Can you work these out from the model? Positions are in its coordinate system, mm. Coordinates: 2 decimals unless noted, no trailing zeros. Order: outer loops, then holes, each group sorted by start corner. A loop starts at its lowest first (then second) coordinate and runs counter-clockwise, first axis right, second up. Notation, with made-up numbers: M -6,23.5 L 48,23.5 A22 ccw 48,58.5 Z; hole C 5.25,-27.5 d1. An arc over 180 degrees is marked long. Answer as a JSON object with one key per item and string values.
Autodesk Inventor part; units mm, degrees
ref_plane "Work Plane1" through (15, -19.5, -83) normal (0, 0, -1) x (0, 1, 0)
ref_plane "YZ Plane" through (0, 0, 0) normal (1, 0, 0) x (0, 1, 0)
ref_plane "XZ Plane" through (0, 0, 0) normal (0, 1, 0) x (-1, 0, 0)
sketch "Sketch2" plane through (0, 0, 0) normal (0, 0, 1) x (1, 0, 0)
  line L0 (12.1829, -15.8377) -> (-1.2308, 1.6)
  line L1 (-1.2308, 1.6) -> (-2.499, 0.6245)
  line L2 (-2.499, 0.6245) -> (10.9147, -16.8133)
  line L3 (10.9147, -16.8133) -> (12.1829, -15.8377)
  line L4 (12, -15.6) -> (100, -15.6)
  line L5 (100, -15.6) -> (100, -14)
  line L6 (12, -14) -> (100, -14)
  line L7 (12, -15.6) -> (12, -14)
  line L8 (0, 0) -> (100, 0)
  line L9 (100, 0) -> (100, 1.6)
  line L10 (0, 1.6) -> (100, 1.6)
  line L11 (0, 0) -> (0, 1.6)
  dimension "d0" = 1.6
  dimension "d1" = 22
ref_plane "Work Plane1" through (15, -19.5, -83) normal (0, 0, -1) x (0, 1, 0)
extrude "Extrusion1" add sketch "Sketch2" against normal blind 100 contours L3 L2 L1 L0
Item 1: I want a section at B-B, the plane y = -13.25. Write out the boundary of the cut face in (x, z).
Answers follow:
{"outline": "M 8.17,-100 L 10.19,-100 L 10.19,0 L 8.17,0 Z"}
Item 2: I want a section at A-A, the plane z = -40. Write out the boundary of the cut face in (x, y), plus the area to 3 significant figures.
Answers follow:
{"outline": "M -2.5,0.62 L 10.91,-16.81 L 12.18,-15.84 L -1.23,1.6 Z", "area": "35.2 mm^2"}
Item 3: I want a section at C-C, the plane x = 4.5. Write out the boundary of the cut face in (y, z).
Answers follow:
{"outline": "M -8.47,-100 L -5.85,-100 L -5.85,0 L -8.47,0 Z"}
Item 4: I'm going to push flat-ended pins straight in: pin 1 (3 mm diameter, centred on y = -4.5, z = -62.5, fed in from +X); pin 2 (2 mm diameter, centred on x = 0.5, z = -51.5, fed in from +Y); pin 3 (1 mm diameter, centred on y = -14, z = -61.5, fed in from +X). Where does each tip first touch, or does it pass through?
Answers follow:
{"pin 1": "stops at x = 4.62", "pin 2": "stops at y = 0.65", "pin 3": "stops at x = 11.15"}
Item 5: Please list where these lines run through material, in increasing order: line 1 (Y direction, x = 8.25, z = -79); line 2 (Y direction, x = 0.75, z = -75); line 3 (X direction, y = -8.5, z = -88).
Answers follow:
{"line 1": "y = -13.35 to -10.72", "line 2": "y = -3.6 to -0.98", "line 3": "x = 4.52 to 6.54"}
